Build history of the part. All positions in model axes, mm. Coordinates: 2 decimals unless noted, no trailing zeros. Loops run counter-clockwise (first coordinate to the right, second up) from the corner with the lowest first, then second, coordinate; pieces in that order, holes last.
(1) Flat gauge pins, fed straight in: P1, Ø3, axis at x = -460, y = 21, coming from the +Z side; P2, Ø5, axis at x = 251.5, z = 12.5, coming from the +Y side; P3, Ø4, axis at x = -730, y = 20, coming from the +Z side. Where does each tip first touch, or does it go through?
(2) Slice it at A-A (x = 404.5). Give the cut face in (y, z).
(3) Slice it at B-B (y = 11). Give the cut face in (x, z), and give its area (3 significant figures).
(4) Wall check: L1, parallel to Z at x = 660, y = 1.95; L2, parallel to Y at x = -688.5, z = 9.25. Give the ranges that are in metal, low to high.
from build123d import *

# Parameters (mm, degrees)
F1_DEPTH = 750
F2_R     = 1
F3_R     = 2.38125
F4_R     = 2.5
F5_DEPTH = 25
F6_SIZE  = 0.5
F7_R     = 2.5
F8_DEPTH = 25
F9_SIZE  = 0.5


with BuildPart() as f1:
    # F0 (on Right) → F1 (new body, symmetric)
    with BuildSketch(Plane.YZ):
        Polygon((0, 25.4), (0, 0), (25.4, 0), (25.4, 4.7625), (4.7625, 4.7625), (4.7625, 25.4), align=None)
    extrude(amount=F1_DEPTH, both=True)

    # F2
    f2_edges = [f1.edges().sort_by_distance(p)[0] for p in [
        (0, 0, 25.4),
        (0, 4.7625, 25.4),
        (0, 0, 0),
        (0, 25.4, 4.7625),
        (0, 25.4, 0),
    ]]
    fillet(f2_edges, radius=F2_R)

    # F3
    f3_edges = [f1.edges().sort_by_distance(p)[0] for p in [
        (0, 4.7625, 4.7625),
    ]]
    fillet(f3_edges, radius=F3_R)

    # F4 (on face) → F5 (cut)
    with BuildSketch(Plane.XY.offset(4.7625)):
        with Locations((-730, 20)):
            Circle(F4_R)
        with Locations((0, 20)):
            Circle(F4_R)
        with Locations((730, 20)):
            Circle(F4_R)
    extrude(amount=-F5_DEPTH, mode=Mode.SUBTRACT)

    # F6
    f6_edges = [f1.edges().sort_by_distance(p)[0] for p in [
        (-732.5, 20, 4.7625),
        (-727.5, 20, 2.38125),
        (-732.5, 20, 0),
        (-2.5, 20, 4.7625),
        (2.5, 20, 2.38125),
        (-2.5, 20, 0),
        (727.5, 20, 4.7625),
        (732.5, 20, 2.38125),
        (727.5, 20, 0),
    ]]
    chamfer(f6_edges, length=F6_SIZE)

    # F7 (on face) → F8 (cut)
    with BuildSketch(Plane.XZ):
        with Locations((-660, 20)):
            Circle(F7_R)
        with Locations((660, 20)):
            Circle(F7_R)
    extrude(amount=-F8_DEPTH, mode=Mode.SUBTRACT)

    # F9
    f9_edges = [f1.edges().sort_by_distance(p)[0] for p in [
        (-662.5, 0, 20),
        (-657.5, 2.38125, 20),
        (-662.5, 4.7625, 20),
        (657.5, 0, 20),
        (662.5, 2.38125, 20),
        (657.5, 4.7625, 20),
    ]]
    chamfer(f9_edges, length=F9_SIZE)


solid = f1.part
Response values:
1. P1: stops at z = 4.76
1. P2: stops at y = 4.76
1. P3: passes through
2. outline: (0, 1) arc R1 ccw to (1, 0) - (24.4, 0) arc R1 ccw to (25.4, 1) - (25.4, 3.76) arc R1 ccw to (24.4, 4.76) - (7.14, 4.76) arc R2.38 cw to (4.76, 7.14) - (4.76, 24.4) arc R1 ccw to (3.76, 25.4) - (1, 25.4) arc R1 ccw to (0, 24.4) - close
3. outline: (-750, 0) - (750, 0) - (750, 4.76) - (-750, 4.76) - close
3. area: 7,140 mm2
4. L1: z = 0 to 17.5, 22.5 to 25.4
4. L2: y = 0 to 4.76
